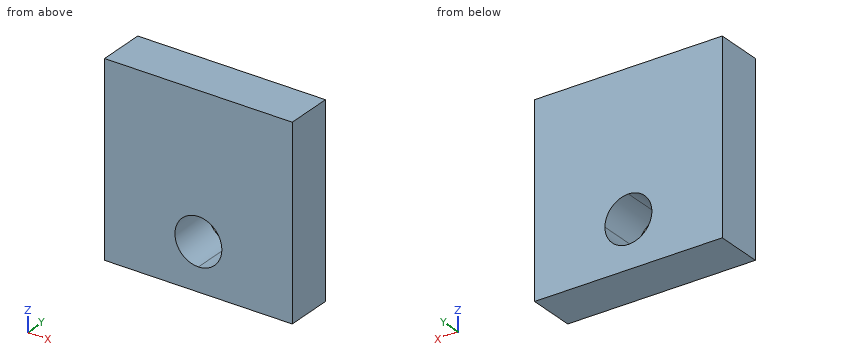
```python
from build123d import *

# Parameters (mm, degrees)
F0_W     = 101.6
F0_H     = 101.6
F1_DEPTH = 25.4
F3_DEPTH = 25.401


with BuildPart() as f1:
    # F0 (on Front) → F1 (new body)
    with BuildSketch(Plane.XZ):
        with Locations((50.8, 50.8)):
            Rectangle(F0_W, F0_H)
    extrude(amount=F1_DEPTH)

    # F2 (on face) → F3 (cut, through all)
    with BuildSketch(Plane.XZ.offset(25.4)):
        with BuildLine():
            ThreePointArc((63.5, 25.4), (59.780256, 34.380256), (50.8, 38.1))
            Line((50.8, 38.1), (50.8, 12.7))
            ThreePointArc((50.8, 12.7), (59.780256, 16.419744), (63.5, 25.4))
        make_face()
        with BuildLine():
            Line((50.8, 12.7), (50.8, 38.1))
            ThreePointArc((50.8, 38.1), (38.1, 25.4), (50.8, 12.7))
        make_face()
    extrude(amount=-F3_DEPTH, mode=Mode.SUBTRACT)


solid = f1.part
```
Design review of the part built by this model. Coordinates are the model's own, in mm. Coordinates: 2 decimals unless noted, no trailing zeros. Write each loop counter-clockwise with the first axis right and the second up, starting at its lowest first coordinate (ties: lowest second). Pieces come first, ordered by that corner, then holes.
1) Add section B-B (z = 21). Write out the cut boundary in (x, y), plus the area to 3 significant figures.
2) To check wall thickness, follow L1, parallel to Z at x = 61.5, y = -16.75; L2, parallel to Z at x = 42, y = -14; L3, parallel to X at y = -8.25, z = 17.5. State the ranges of each line that lie inside material, in increasing order.
3) Add section A-A (y = -4). Write out the cut boundary in (x, z), plus the area to 3 significant figures.
4) Insertion check: pin 1 (2 mm diameter, centred on x = 59.5, z = 40, fed in from +Y). The pin has a flat end and moves straight along its axis. Give the tip position at first contact, or say it passes through.
Check result:
1. outline: (0, -25.4) - (38.89, -25.4) - (38.89, 0) - (0, 0) - close; (62.71, -25.4) - (101.6, -25.4) - (101.6, 0) - (62.71, 0) - close
1. area: 1,980 mm2
2. L1: z = 0 to 18.56, 32.24 to 101.6
2. L2: z = 0 to 16.24, 34.56 to 101.6
2. L3: x = 0 to 40.86, 60.74 to 101.6
3. outline: (0, 0) - (101.6, 0) - (101.6, 101.6) - (0, 101.6) - close; hole circle Ø25.4 at (50.8, 25.4)
3. area: 9,820 mm2
4. pin 1: stops at y = 0
